Geometry check sheet. Reference: the model listing, model coordinates, mm. Round coordinates to 2 decimals unless told otherwise and drop trailing zeros. Write each loop counter-clockwise with the first axis right and the second up, starting at its lowest first coordinate (ties: lowest second). Pieces come first, ordered by that corner, then holes. Notation, with made-up numbers: M -5.75,5 L 40.25,5 A12 ccw 40.25,26 Z; hole C 88,3 d11. An arc over 180 degrees is marked long. Use a Markdown table: item, result.
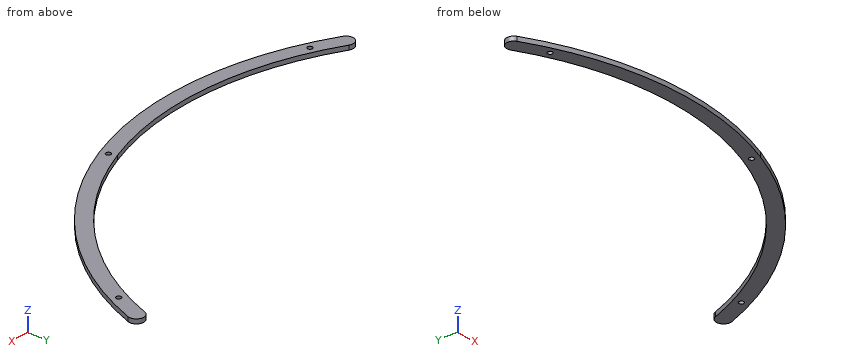
```python
from build123d import *

# Parameters (mm, degrees)
PAD014_DEPTH                        = 3
SKETCH055_R                         = 1.65
POCKET019_DEPTH                     = 364.282338
POCKET019_DEPTH_BACK                = 367.282338
BODY001003005003003_PLACEMENT_ANGLE = 60
CLONE_PLACEMENT_ANGLE               = 141


with BuildPart() as part:
    # Sketch052 → Pad014 (new body)
    with BuildSketch(Plane.XY):
        with BuildLine():
            ThreePointArc((152.959511, 127.101705), (84.480895, 180.040089), (0, 198.875477))
            Line((0, 198.875477), (0, 208.875477))
            ThreePointArc((160.650731, 133.492724), (88.728824, 189.092995), (0, 208.875477))
            ThreePointArc((152.959511, 127.101705), (160.000631, 126.451604), (160.650731, 133.492724))
        make_face()
    pad014 = extrude(amount=PAD014_DEPTH)

    # Sketch055 → Pocket019 (cut, two sides)
    with BuildSketch(Plane.XY) as pocket019_sk:
        with Locations((143.11, 145.205847)):
            Circle(SKETCH055_R)
        with BuildLine():
            Line((0, 202.225477), (0, 205.525477))
            ThreePointArc((0, 202.225477), (1.65, 203.875477), (0, 205.525477))
        make_face()
    pocket019 = extrude(amount=-POCKET019_DEPTH, mode=Mode.SUBTRACT) + extrude(pocket019_sk.sketch, amount=POCKET019_DEPTH_BACK, mode=Mode.SUBTRACT)

    # Mirrored019: Pad014, Pocket019 across Sketch052 V_Axis
    add(pad014.mirror(Plane(origin=(0, 0, 0), x_dir=(0, 0, 1), z_dir=(1, 0, 0))))
    add(pocket019.mirror(Plane(origin=(0, 0, 0), x_dir=(0, 0, 1), z_dir=(1, 0, 0))), mode=Mode.SUBTRACT)


with BuildPart() as part_1:
    # Body001003005003003 placement: moved
    add(part.part.rotate(Axis((0, 0, 0), (0, 0, 1)), BODY001003005003003_PLACEMENT_ANGLE))


with BuildPart() as part_2:
    # Clone placement: moved
    add(part_1.part.moved(Location((1296, 766, 0))).rotate(Axis((1296, 766, 0), (0, 0, 1)), CLONE_PLACEMENT_ANGLE))


solid = part_2.part
```
Item 1: Go/stop test with flat-tipped pins: pin 1 (1.5 mm diameter, centred on y = 687, z = 2, fed in from +X); pin 2 (5.5 mm diameter, centred on x = 1481.64, y = 681.72, fed in from -Z). Record where each tip stops, or that it passes through.
Outcome:
| item | result |
|---|---|
| pin 1 | stops at x = 1489.66 |
| pin 2 | stops at z = 0 |
Item 2: Cross-section at C-C, the plane x = 1342. Record the cut outline in (y, z), and give its area (3 significant figures).
Outcome:
| item | result |
|---|---|
| outline | M 562.25,0 L 572.52,0 L 572.52,3 L 562.25,3 Z |
| area | 30.8 mm2 |
Item 3: Cross-section at B-B, the plane y = 642. Record the cut outline in (x, z), and give its area (3 significant figures).
Outcome:
| item | result |
|---|---|
| outline | M 1451.48,0 L 1464.09,0 L 1464.09,3 L 1451.48,3 Z |
| area | 37.8 mm2 |
Item 4: Cross-section at A-A, the plane z = 1.55. Record the cut outline in (x, y), and give its area (3 significant figures).
Outcome:
| item | result |
|---|---|
| outline | M 1193.86,583.8 A208.88 ccw 1370.85,571 A208.88 ccw 1493.82,698.95 A5 ccw 1484.35,702.16 A198.88 cw 1367.27,580.33 A198.88 cw 1198.75,592.52 A5 ccw Z; hole C 1214.43,579.15 d3.3; hole C 1369.06,575.67 d3.3; hole C 1481.64,681.72 d3.3 |
| area | 3,630 mm2 |
Item 5: Material ranges on line 1 along X through (y, z) = (681.5, 1.7); line 2 along Y through (x, z) = (1213, 2.2); line 3 along X through (y, z) = (584, 0.7) (3 decimals), recorded low to high. Write a range as from..to.
Outcome:
| item | result |
|---|---|
| line 1 | x = 1476.03..1480.01, 1483.28..1487.02 |
| line 2 | y = 574.32..578.33, 579.97..585.27 |
| line 3 | x = 1193.535..1215.829, 1376.171..1398.494 |
